Autodesk Fusion 360 part; units mm, degrees
sketch "Sketch1" plane through (0, 0, 0) normal (0, 0, 1) x (1, 0, 0)
  line L0 (0, 0) -> (150, 0)
  line L1 (150, 0) -> (150, 150)
  line L2 (150, 150) -> (0, 150)
  line L3 (0, 150) -> (0, 0)
  dimension "d1" = 150
  dimension "d2" = 150
extrude "Extrude2" add sketch "Sketch1" along normal blind 10
sketch "Sketch3" plane through (0, 0, 10) normal (0, 0, 1) x (-1, 0, 0)
  line L0 (0, -150) -> (0, 0)
  line L1 (0, 0) -> (-150, 0)
  line L2 (-150, 0) -> (-150, -150)
  line L3 (-150, -150) -> (0, -150)
  circle A0 centre (-15, -135) radius 10
  dimension "d7" = 20
  dimension "d8" = 15
  dimension "d9" = 15
extrude "Extrude3" cut sketch "Sketch3" against normal blind 5 contours A0
pattern_linear "R-Pattern1" count 6 spacing 24 along (1, 0, 0) count 6 spacing 24 along (0, -1, 0) of "Extrude3"
Part model, mm, in its own coordinate system. Coordinates: 2 decimals unless noted, no trailing zeros. Loops run counter-clockwise (first coordinate to the right, second up) from the corner with the lowest first, then second, coordinate; pieces in that order, holes last. Notation, with made-up numbers: (39.5, 49.25) - (52.5, 49.25) arc R21 ccw to (52.5, 76.25) - close; hole circle Ø8 at (-40, -34.75). An arc over 180 degrees is marked (long way). Write item = value, one per line. Start each with the question number.
Item 1: Wall check: L1, parallel to Z at x = 53.5, y = 135.5. Give the ranges that are in metal, low to high. Write a range as from..to.
Item 2: Cut at A-A, the plane y = 15. Give the cut face in (x, z), and give its area (3 significant figures).
Item 3: Mould opens along Y. For faces 1 (the flat face through (150, 74, 5)), 2 (the cylindrical face through (5.46, 12, 7.54)) say: released by +Y, released by -Y, zero draft, split by the parting line, or undercut.
Item 4: Flat gauge pins, fed straight in: pin 1 Ø5 at (x, y) = (50, 120.5) entering from -Z; pin 2 Ø12 at (x, y) = (87, 63) entering from +Z. Where does each tip first touch, or does it go through?
Item 5: Cut at C-C, the plane z = 6.5. State how many separate pieces and enclosed holes the cut face has, and give its area (3 significant figures).
The answers:
q1.L1 = 0..5
q2.outline = (0, 0) - (150, 0) - (150, 10) - (145, 10) - (145, 5) - (125, 5) - (125, 10) - (121, 10) - (121, 5) - (101, 5) - (101, 10) - (97, 10) - (97, 5) - (77, 5) - (77, 10) - (73, 10) - (73, 5) - (53, 5) - (53, 10) - (49, 10) - (49, 5) - (29, 5) - (29, 10) - (25, 10) - (25, 5) - (5, 5) - (5, 10) - (0, 10) - close
q2.area = 900 mm2
q3.face_1 = zero draft
q3.face_2 = undercut
q4.pin_1 = 0
q4.pin_2 = 5
q5.separate_pieces = 1
q5.enclosed_holes = 36
q5.area = 11,200 mm2
